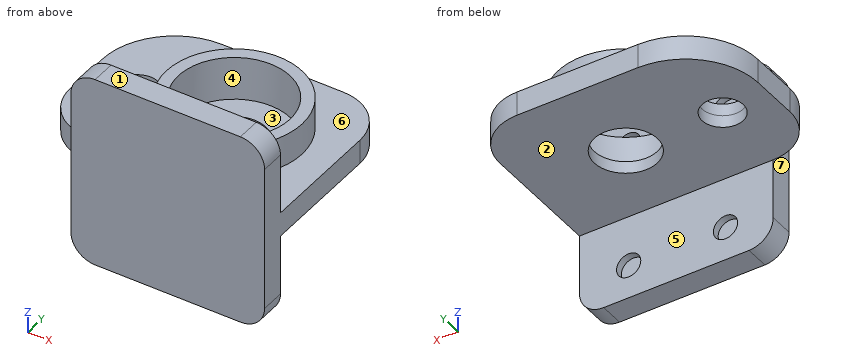
from build123d import *

# Parameters (mm, degrees)
F0_W      = 20
F0_H      = 5
F1_DEPTH  = 20
F1_FACE_W = 40
F1_FACE_H = 5
F2_DEPTH  = 20
F0_R      = 14
F0_R_2    = 11.5
F3_DEPTH  = 9
F0_R_3    = 4.25
F4_DEPTH  = 2.5
F0_R_4    = 6.5
F5_DEPTH  = 2.5
F6_R      = 15
F6_2_R    = 15
F7_R      = 10
F7_2_R    = 10
F8_R      = 10
F8_2_R    = 10
F9_R      = 5
F11_R     = 2.5
F12_DEPTH = 1.5


with BuildPart() as f1:
    # F0 (on Top) → F1 (new body)
    with BuildSketch(Plane.XY):
        with Locations((-9.850006, -18.65)):
            Rectangle(F0_W, F0_H)
        with Locations((10.149994, -18.65)):
            Rectangle(F0_W, F0_H)
    extrude(amount=F1_DEPTH)

    # F1_face (on face) → F2 (join)
    with BuildSketch(Plane(origin=(0.149994, -18.65, 0), x_dir=(1, 0, 0), z_dir=(0, 0, -1))):
        Rectangle(F1_FACE_W, F1_FACE_H)
    extrude(amount=F2_DEPTH)

    # F9
    f9_edges = [f1.edges().sort_by_distance(p)[0] for p in [
        (-19.850006, -18.65, 20),
        (20.149994, -18.65, 20),
        (20.149994, -18.65, -20),
        (-19.850006, -18.65, -20),
    ]]
    fillet(f9_edges, radius=F9_R)


with BuildPart() as f3:
    # F0 (on Top) → F3 (new body)
    with BuildSketch(Plane.XY):
        Circle(F0_R)
        Circle(F0_R_2, mode=Mode.SUBTRACT)
    extrude(amount=F3_DEPTH)


with BuildPart() as f4:
    # F0 (on Top) → F4 (new body)
    with BuildSketch(Plane.XY):
        Polygon((-19.850006, -16.15), (0.149994, -16.15), (20.149994, -16.15), (20.149994, 18.85), (-29.850006, 18.85), (-29.850006, -16.15), align=None)
        with Locations((-20, 0)):
            Circle(F0_R_3, mode=Mode.SUBTRACT)
        Circle(F0_R, mode=Mode.SUBTRACT)
        Circle(F0_R)
        Circle(F0_R_2, mode=Mode.SUBTRACT)
    extrude(amount=F4_DEPTH)

    # F6#2
    f6_2_edges = [f4.edges().sort_by_distance(p)[0] for p in [
        (-29.850006, 18.85, 1.25),
    ]]
    fillet(f6_2_edges, radius=F6_2_R)

    # F7#2
    f7_2_edges = [f4.edges().sort_by_distance(p)[0] for p in [
        (20.149994, 18.85, 1.25),
    ]]
    fillet(f7_2_edges, radius=F7_2_R)

    # F8#2
    f8_2_edges = [f4.edges().sort_by_distance(p)[0] for p in [
        (-29.850006, -16.15, 1.25),
    ]]
    fillet(f8_2_edges, radius=F8_2_R)


with BuildPart() as f5:
    # F0 (on Top) → F5 (new body)
    with BuildSketch(Plane.XY):
        Polygon((-19.850006, -16.15), (0.149994, -16.15), (20.149994, -16.15), (20.149994, 18.85), (-29.850006, 18.85), (-29.850006, -16.15), align=None)
        with Locations((-20, 0)):
            Circle(F0_R_3, mode=Mode.SUBTRACT)
        Circle(F0_R, mode=Mode.SUBTRACT)
        Circle(F0_R)
        Circle(F0_R_2, mode=Mode.SUBTRACT)
        Circle(F0_R_2)
        Circle(F0_R_4, mode=Mode.SUBTRACT)
    extrude(amount=-F5_DEPTH)

    # F6
    f6_edges = [f5.edges().sort_by_distance(p)[0] for p in [
        (-29.850006, 18.85, -1.25),
    ]]
    fillet(f6_edges, radius=F6_R)

    # F7
    f7_edges = [f5.edges().sort_by_distance(p)[0] for p in [
        (20.149994, 18.85, -1.25),
    ]]
    fillet(f7_edges, radius=F7_R)

    # F8
    f8_edges = [f5.edges().sort_by_distance(p)[0] for p in [
        (-29.850006, -16.15, -1.25),
    ]]
    fillet(f8_edges, radius=F8_R)


with BuildPart() as f1_1:
    add(f1.part)

    # F10: union F3, F4, F5
    add(f3.part)
    add(f4.part)
    add(f5.part)

    # F11 (on face) → F12 (cut)
    with BuildSketch(Plane(origin=(0, -16.15, 0), x_dir=(-1, 0, 0), z_dir=(0, 1, 0))):
        with Locations((-10, 13)):
            Circle(F11_R)
        with Locations((10, 13)):
            Circle(F11_R)
        with Locations((-10, -13)):
            Circle(F11_R)
        with Locations((10, -13)):
            Circle(F11_R)
    extrude(amount=-F12_DEPTH, mode=Mode.SUBTRACT)


solid = f1_1.part
Verification items for the finished model (mm, model axes). Face numbers are marked on the shaded views. A direction names the side the tool comes from. Round coordinates to 2 decimals unless told otherwise and drop trailing zeros. Order: outer loops, then holes, each group sorted by start corner. A loop starts at its lowest first (then second) coordinate and runs counter-clockwise, first axis right, second up.
1. Release check for a two-part mould opening along Y. For the marked faces 4, 5, 6 and 7 record: +Y half, -Y half, draft (parallel to the pull), parting line (faces both ways), or undercut.
Final values:
face 4: undercut
face 5: +Y half
face 6: undercut
face 7: draft
2. Section check B-B on y = 0. Record the cut outline in (x, z).
Final values:
outline: (-29.85, -2.5) - (-24.25, -2.5) - (-24.25, 2.5) - (-29.85, 2.5) - close; (-15.75, -2.5) - (-6.5, -2.5) - (-6.5, 0) - (-11.5, 0) - (-11.5, 9) - (-14, 9) - (-14, 2.5) - (-15.75, 2.5) - close; (6.5, -2.5) - (20.15, -2.5) - (20.15, 2.5) - (14, 2.5) - (14, 9) - (11.5, 9) - (11.5, 0) - (6.5, 0) - close
3. Section check C-C on z = -13. Record the cut outline in (x, y).
Final values:
outline: (-19.85, -21.15) - (20.15, -21.15) - (20.15, -16.15) - (12.5, -16.15) - (12.5, -17.65) - (7.5, -17.65) - (7.5, -16.15) - (-7.5, -16.15) - (-7.5, -17.65) - (-12.5, -17.65) - (-12.5, -16.15) - (-19.85, -16.15) - close
4. Thickness scan on L1, parallel to Z at x = -10, y = -17.25; L2, parallel to Y at x = 0, z = -0.8; L3, parallel to Y at x = -3.5, z = 8. Record the ranges inside material, lowest first.
Final values:
L1: z = -20 to -15.5, -10.5 to 10.5, 15.5 to 20
L2: y = -21.15 to -6.5, 6.5 to 18.85
L3: y = -21.15 to -16.15, -13.56 to -10.95, 10.95 to 13.56
5. Section check A-A on x = 0. Record the cut outline in (y, z).
Final values:
outline: (-21.15, -20) - (-16.15, -20) - (-16.15, -2.5) - (-6.5, -2.5) - (-6.5, 0) - (-11.5, 0) - (-11.5, 9) - (-14, 9) - (-14, 2.5) - (-16.15, 2.5) - (-16.15, 20) - (-21.15, 20) - close; (6.5, -2.5) - (18.85, -2.5) - (18.85, 2.5) - (14, 2.5) - (14, 9) - (11.5, 9) - (11.5, 0) - (6.5, 0) - close
6. Section check D-D on y = -5. Record the cut outline in (x, z).
Final values:
outline: (-29.85, -2.5) - (-4.15, -2.5) - (-4.15, 0) - (-10.36, 0) - (-10.36, 9) - (-13.08, 9) - (-13.08, 2.5) - (-29.85, 2.5) - close; (4.15, -2.5) - (20.15, -2.5) - (20.15, 2.5) - (13.08, 2.5) - (13.08, 9) - (10.36, 9) - (10.36, 0) - (4.15, 0) - close
7. Go/stop test with flat-tipped pins: P1, Ø10, axis at x = -15.5, y = 10.5, coming from the +Z side; P2, Ø15, axis at x = 0, y = 0, coming from the -Z side; P3, Ø6, axis at x = -10, z = -13, coming from the +Y side. Record where each tip stops, or that it passes through.
Final values:
P1: stops at z = 9
P2: stops at z = -2.5
P3: stops at y = -16.15
8. Access from +Z, -Z, +X, -X, +Y, -Y to the whole of each face (thin tool, end or side, straight path). Record for the marked faces 1, 2 and 3.
Final values:
face 1: +Z, +X, -X, +Y, -Y
face 2: -Z, +X, -X, +Y
face 3: +Z
